Autodesk Inventor part; units mm, degrees
ref_plane "YZ Plane" through (0, 0, 0) normal (1, 0, 0) x (0, 1, 0)
ref_plane "XZ Plane" through (0, 0, 0) normal (0, 1, 0) x (-1, 0, 0)
ref_plane "XY Plane" through (0, 0, 0) normal (0, 0, 1) x (1, 0, 0)
sketch "Sketch1" plane through (0, 0, 0) normal (0, 0, 1) x (1, 0, 0)
  line L0 (-15.25, 18) -> (15.25, 18)
  line L1 (15.25, 18) -> (15.25, -18)
  line L2 (15.25, -18) -> (-15.25, -18)
  line L3 (-15.25, -18) -> (-15.25, 18)
  point P0 (0, 0)
  dimension "d0" = 30.5
  dimension "d1" = 36
  dimension "d2" = 18
  dimension "d3" = 15.25
extrude "Extrusion1" add sketch "Sketch1" along normal blind 5.5
sketch "Sketch2" plane through (-15.25, 18, 0) normal (0, 1, 0) x (1, 0, 0)
  line L0 (30.5, 0) -> (30.5, -8.35)
  line L1 (30.5, -8.35) -> (70.5, -8.35)
  line L2 (70.5, 11.65) -> (70.5, -8.35)
  line L3 (0, 11.65) -> (70.5, 11.65)
  line L4 (0, 11.65) -> (0, 0.5)
  line L5 (0, 0.5) -> (9.7766, 0.5)
  arc A0 (19.2498, 0) -> (9.7766, 0.5) centre (14.5, 0) ccw
  line L6 (19.2498, 0) -> (30.5, 0)
  circle A1 centre (40.5, 1.65) radius 0.847
  circle A2 centre (62.5, 1.65) radius 0.847
  circle A3 centre (54.5, 1.65) radius 4
  circle A4 centre (14.5, 0) radius 4.7498
  point P0 (15.25, 0)
extrude "Extrusion2" cut sketch "Sketch2" against normal through all contours A4 A0
sketch "Sketch3" plane through (0, 0, 5.5) normal (0, 0, 1) x (1, 0, 0)
  circle A0 centre (-11.25, 12) radius 1.0065
  circle A1 centre (-11.25, 0) radius 1.0065
  circle A2 centre (-11.25, -12) radius 1.0065
  circle A3 centre (9.7764, 12) radius 1.0065
  circle A4 centre (9.7764, 0) radius 1.0065
  circle A5 centre (9.7764, -12) radius 1.0065
  point P0 (0, 0)
hole "CBore for M2.5 screw" at (-11.25, -12, 5.5) at (-11.25, 0, 5.5) at (-11.25, 12, 5.5) at (9.7764, -12, 5.5) at (9.7764, 0, 5.5) at (9.7764, 12, 5.5) direction (0, 0, -1) diameter 2.9 end through all counterbore diameter 5.5 counterbore depth 2.5
sketch "Sketch4" plane through (0, 0, 0) normal (0, 0, -1) x (-1, 0, 0)
  circle A0 centre (11.25, 0) radius 1.45
  circle A1 centre (11.25, -12) radius 1.45
  circle A2 centre (11.25, 12) radius 1.45
  line L0 (5.4998, 18) -> (5.4998, -18)
  line L1 (5.4998, -18) -> (15.25, -18)
  line L2 (15.25, -18) -> (15.25, 18)
  line L3 (15.25, 18) -> (5.4998, 18)
  line L4 (15.25, -18) -> (4.4998, -18)
  line L5 (4.4998, -18) -> (4.4998, 18)
  line L6 (4.4998, 18) -> (15.25, 18)
  line L7 (15.25, 18) -> (15.25, -18)
  point P0 (0, 0)
  dimension "d17" = 1
extrude "Extrusion3" cut sketch "Sketch4" against normal blind 0.5
properties part number "J007580" material "ALUMINUM, 6061-T651"
Work out the finished part from the listing and answer in its coordinate system (mm). A direction names the side the tool comes from. Round coordinates to 2 decimals unless told otherwise and drop trailing zeros. Loops run counter-clockwise (first coordinate to the right, second up) from the corner with the lowest first, then second, coordinate; pieces in that order, holes last. Notation, with made-up numbers: M -12.75,49.25 L 15.25,49.25 A9 cw 15.25,56.25 Z; hole C 11,68 d4. An arc over 180 degrees is marked long. Use CSV: the item, a comma, the result in double quotes.
Q1. Section A-A, the plane z = 3.6 is taken. Determine the outline of the cut face in (x, y), then the cut area to 3 significant figures.
Determined:
outline,"M -15.25,-18 L -3.85,-18 L -3.85,18 L -15.25,18 Z; M 2.35,-18 L 15.25,-18 L 15.25,18 L 2.35,18 Z; hole C -11.25,-12 d5.5; hole C -11.25,0 d5.5; hole C -11.25,12 d5.5; hole C 9.78,-12 d5.5; hole C 9.78,0 d5.5; hole C 9.78,12 d5.5"
area,"732 mm2"
Q2. A tool of negligible diameter and unlimited length cuts with its end or side. For faces 4 (the flat face through (-9, 0, 0.5)), 5 (the cylindrical face through (-14, 0, 4)), 6 (the flat face through (-15.25, 0, 3)), from which of +Z, -Z, +X, -X, +Y, -Y can it reach the whole face along a straight path? Write none if from no direction.
Determined:
face 4,"-Z, -X, +Y, -Y"
face 5,"+Z"
face 6,"+Z, -Z, -X, +Y, -Y"
Q3. Section D-D, the plane x = 7.5 is taken. Determine the outline of the cut face in (y, z), then the cut area to 3 significant figures.
Determined:
outline,"M -18,0 L 18,0 L 18,5.5 L 13.54,5.5 L 13.54,3 L 10.46,3 L 10.46,5.5 L 1.54,5.5 L 1.54,3 L -1.54,3 L -1.54,5.5 L -10.46,5.5 L -10.46,3 L -13.54,3 L -13.54,5.5 L -18,5.5 Z"
area,"175 mm2"
Q4. Section C-C, the plane y = -12 is taken. Determine the outline of the cut face in (x, z).
Determined:
outline,"M -15.25,0.5 L -12.7,0.5 L -12.7,3 L -14,3 L -14,5.5 L -15.25,5.5 Z; M -9.8,0.5 L -5.47,0.5 A4.75 cw 4,0 L 8.33,0 L 8.33,3 L 7.03,3 L 7.03,5.5 L -8.5,5.5 L -8.5,3 L -9.8,3 Z; M 11.23,0 L 15.25,0 L 15.25,5.5 L 12.53,5.5 L 12.53,3 L 11.23,3 Z"
Q5. The mould has two halves that part along X. Classify faces 1 (the flat face through (0, -18, 5)), 2 (the flat face through (15.25, 0, 3)), 3 (the cylindrical face through (-10.37, 13.15, 1.73)): pulls with the +X half, pulls with the -X half, needs draft (parallel to the pull), parting line crosses it, or undercut.
Determined:
face 1,"needs draft"
face 2,"pulls with the +X half"
face 3,"undercut"
Q6. Each of these flat-tipped pins is pushed along its axis until it touches: pin 1 (3 mm diameter, centred on x = -12, y = 0, fed in from +Z); pin 2 (1.5 mm diameter, centred on x = -1, y = -7, fed in from -Z); pin 3 (2.5 mm diameter, centred on x = 9.78, y = 0, fed in from +Z); pin 4 (3.5 mm diameter, centred on x = -11.25, y = 12, fed in from -Z). Where does it stop, or does it pass through?
Determined:
pin 1,"z = 3"
pin 2,"z = 4.64"
pin 3,"through"
pin 4,"z = 0.5"
Q7. Consider L1, parallel to Y at x = -11.25, z = 3.5; L2, parallel to Y at x = -11.25, z = 1.8; L3, parallel to X at y = 12, z = 1.9. Determine where each line is inside the solid, lowest interval first.
Determined:
L1,"-18 to -14.75, -9.25 to -2.75, 2.75 to 9.25, 14.75 to 18"
L2,"-18 to -13.45, -10.55 to -1.45, 1.45 to 10.55, 13.45 to 18"
L3,"-15.25 to -12.7, -9.8 to -5.1, 3.6 to 8.33, 11.23 to 15.25"
Q8. Section B-B, the plane x = -11.25 is taken. Determine the outline of the cut face in (y, z).
Determined:
outline,"M -18,0.5 L -13.45,0.5 L -13.45,3 L -14.75,3 L -14.75,5.5 L -18,5.5 Z; M -10.55,0.5 L -1.45,0.5 L -1.45,3 L -2.75,3 L -2.75,5.5 L -9.25,5.5 L -9.25,3 L -10.55,3 Z; M 1.45,0.5 L 10.55,0.5 L 10.55,3 L 9.25,3 L 9.25,5.5 L 2.75,5.5 L 2.75,3 L 1.45,3 Z; M 13.45,0.5 L 18,0.5 L 18,5.5 L 14.75,5.5 L 14.75,3 L 13.45,3 Z"
